Study the drawing (mm; zero at the part's minimum x, y, z) and answer. A direction names the side the tool comes from. Round coordinates to 2 decimals unless told otherwise and drop trailing zeros. Loops run counter-clockwise (first coordinate to the right, second up) from the corner with the lowest first, then second, coordinate; pieces in that order, holes last. Notation, with made-up numbers: (-30, 89.25) -> (-14, 89.25) arc R29 ccw to (-14, 115.25) -> close; hole circle Ø11 at (5, -11). An arc over 180 degrees is marked (long way). Use one line per item in the form item = value.
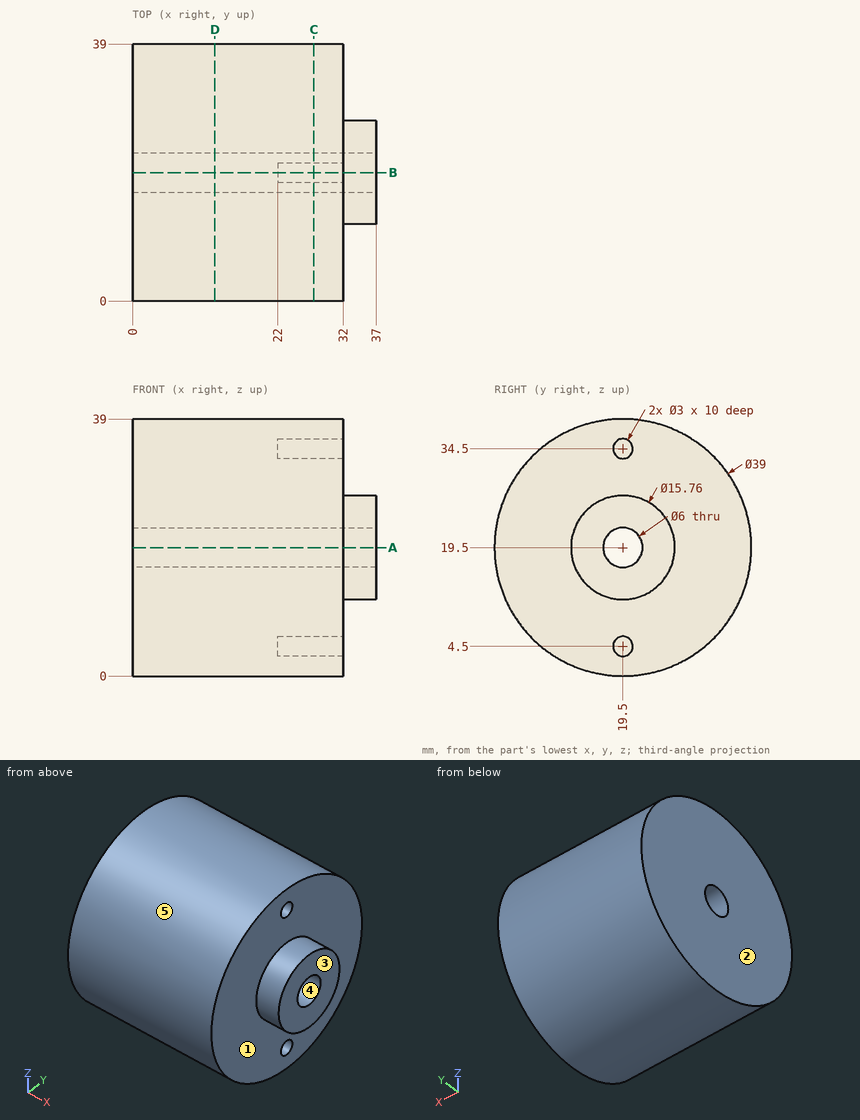
(1) For the marked faces 1 and 2, determine the directions among +Z, -Z, +X, -X, +Y, -Y from which every point of the face is accessible in a straight line to the end or side of a thin tool.
Completed:
face_1 = +X
face_2 = +Z, -Z, -X, +Y, -Y
(2) For a pull along Y with two mould halves and no side action, classify the marked faces 3, 4 and 5 as +Y half, -Y half, draft (parallel to the pull), parting line (faces both ways), or undercut.
Completed:
face_3 = draft
face_4 = undercut
face_5 = parting line
(3) Find section C-C, the plane x = 27.5. Write down the section's boundary in (y, z), then the cut area to 3 significant figures.
Completed:
outline = circle Ø39 at (19.5, 19.5); hole circle Ø6 at (19.5, 19.5); hole circle Ø3 at (19.5, 4.5); hole circle Ø3 at (19.5, 34.5)
area = 1,150 mm2
(4) Find section A-A, the plane z = 19.5. Write down the section's boundary in (x, y).
Completed:
outline = (0, 0) -> (32, 0) -> (32, 11.62) -> (37, 11.62) -> (37, 16.5) -> (0, 16.5) -> close; (0, 22.5) -> (37, 22.5) -> (37, 27.38) -> (32, 27.38) -> (32, 39) -> (0, 39) -> close
(5) Given P1, Ø4, axis at y = 19.5, z = 4.5, coming from the +X side; P2, Ø3, axis at x = 8.5, y = 25, coming from the -Z side; P3, Ø12, axis at x = 33, z = 32.5, coming from the -Y side, each flat-ended and moving along its own axis, determine where each tip first touches the part or whether it passes through.
Completed:
P1 = 32
P2 = 0.41
P3 = 1.33
(6) Consider L1, parallel to Z at x = 27, y = 19; L2, parallel to X at y = 11, z = 22; L3, parallel to Z at x = 29, y = 21.5. Determine where each line is inside the solid, lowest interval first.
Completed:
L1 = 0.01 to 3.09, 5.91 to 16.54, 22.46 to 33.09, 35.91 to 38.99
L2 = 0 to 32
L3 = 0.1 to 17.26, 21.74 to 38.9
(7) Find section B-B, the plane y = 19.5. Write down the section's boundary in (x, z).
Completed:
outline = (0, 0) -> (32, 0) -> (32, 3) -> (22, 3) -> (22, 6) -> (32, 6) -> (32, 11.62) -> (37, 11.62) -> (37, 16.5) -> (0, 16.5) -> close; (0, 22.5) -> (37, 22.5) -> (37, 27.38) -> (32, 27.38) -> (32, 33) -> (22, 33) -> (22, 36) -> (32, 36) -> (32, 39) -> (0, 39) -> close
(8) Find section D-D, the plane x = 12.5. Write down the section's boundary in (y, z).
Completed:
outline = circle Ø39 at (19.5, 19.5); hole circle Ø6 at (19.5, 19.5)
